Check sheet for the modelled part. Datum: model origin and axes. Units: mm. A direction names the side the tool comes from. Round coordinates to 2 decimals unless told otherwise and drop trailing zeros. Order: outer loops, then holes, each group sorted by start corner. A loop starts at its lowest first (then second) coordinate and runs counter-clockwise, first axis right, second up. Notation, with made-up numbers: (-40, -7) -> (7, -7) arc R19 cw to (7, 5) -> close; hole circle Ø2 at (86, 60.25). An arc over 180 degrees is marked (long way). Answer in a Markdown table with one row per item. Add a question column.
1. Access from +Z, -Z, +X, -X, +Y, -Y to the whole of each face (thin tool, end or side, straight path). Record for faces 5 (the flat face through (10, -120, 4)), 6 (the cylindrical face through (29.62, -151.84, 6.52)), 7 (the flat face through (40, -150, 4)).
2. Sectioned sample at C-C, the plane z = 1.25. Record the boundary of the cut face in (x, y), then the cut area to 3 significant figures.
3. Sectioned sample at A-A, the plane y = -145. Record the boundary of the cut face in (x, z), then the cut area to 3 significant figures.
4. Sectioned sample at B-B, the plane x = 32. Record the boundary of the cut face in (y, z).
5. Material ranges on L1, parallel to Y at x = 0, z = 5.7; L2, parallel to Y at x = 0, z = 3.05; L3, parallel to X at y = -125, z = 4.05, recorded low to high. Write a range as from..to.
6. Depth check by flat-ended pin: P1, Ø1.8, axis at x = -1, y = -145, coming from the +Z side; P2, Ø2.5, axis at y = -119.5, z = 3.5, coming from the +X side; P3, Ø3.5, axis at x = 0, y = -145, coming from the -Z side; P4, Ø4, axis at x = 29.5, z = 2.5, coming from the +Y side. Enter the tip coordinate at first touch or a pass-through.
7. Sectioned sample at D-D, the plane z = 6.75. Record the boundary of the cut face in (x, y), then the cut area to 3 significant figures.
8. Draft check along X on faces 1 (the flat face through (-10, -130, 4)), 2 (the flat face through (19.3, -151.3, 5)), 3 (the cylindrical face through (-0.35, -146.56, 2.46)), 4 (the flat face through (10, -140, 0)). Enter one of: +X half, -X half, draft (parallel to the pull), parting line (faces both ways), or undercut.
```python
from build123d import *

# Parameters (mm, degrees)
SKETCH_1_R          = 1.6
EXTRUDE_1_DEPTH     = 8
SKETCH_2_R          = 3
CUT_EXTRUDE_1_DEPTH = 3
FILLET_1_R          = 10


with BuildPart() as part:
    # 草图1 → 凸台-拉伸1 (new body)
    with BuildSketch(Plane.XY):
        Polygon((-10, -110), (10, -110), (10, -140.028839027), (40, -140.028839027), (40, -160), (-10, -160), align=None)
        with Locations((0, -125)):
            Circle(SKETCH_1_R, mode=Mode.SUBTRACT)
        with Locations((0, -145)):
            Circle(SKETCH_1_R, mode=Mode.SUBTRACT)
        with Locations((18, -150.014419513)):
            Circle(SKETCH_1_R, mode=Mode.SUBTRACT)
        with Locations((32, -150.014419513)):
            Circle(SKETCH_1_R, mode=Mode.SUBTRACT)
    extrude(amount=EXTRUDE_1_DEPTH)

    # 草图2 → 切除-拉伸1 (cut)
    with BuildSketch(Plane.XY.offset(8)):
        with Locations((32, -150.014419513)):
            Circle(SKETCH_2_R)
        with Locations((18, -150.014419513)):
            Circle(SKETCH_2_R)
        with Locations((0, -145)):
            Circle(SKETCH_2_R)
        with Locations((0, -125)):
            Circle(SKETCH_2_R)
    extrude(amount=-CUT_EXTRUDE_1_DEPTH, mode=Mode.SUBTRACT)

    # 圆角1
    fillet_1_edges = [part.edges().sort_by_distance(p)[0] for p in [
        (10, -140.028839027, 4),
        (-10, -160, 4),
    ]]
    fillet(fillet_1_edges, radius=FILLET_1_R)


solid = part.part
```
Answer key:
| question | item | result |
|---|---|---|
| 1 | face 5 | +Z, -Z, +X, +Y |
| 1 | face 6 | +Z |
| 1 | face 7 | +Z, -Z, +X, +Y, -Y |
| 2 | outline | (-10, -150) arc R10 ccw to (0, -160) -> (40, -160) -> (40, -140.03) -> (20, -140.03) arc R10 cw to (10, -130.03) -> (10, -110) -> (-10, -110) -> close; hole circle Ø3.2 at (0, -145); hole circle Ø3.2 at (0, -125); hole circle Ø3.2 at (18, -150.01); hole circle Ø3.2 at (32, -150.01) |
| 2 | area | 1,570 mm² |
| 3 | outline | (-10, 0) -> (-1.6, 0) -> (-1.6, 5) -> (-3, 5) -> (-3, 8) -> (-10, 8) -> close; (1.6, 0) -> (40, 0) -> (40, 8) -> (3, 8) -> (3, 5) -> (1.6, 5) -> close |
| 3 | area | 366 mm² |
| 4 | outline | (-160, 0) -> (-151.61, 0) -> (-151.61, 5) -> (-153.01, 5) -> (-153.01, 8) -> (-160, 8) -> close; (-148.41, 0) -> (-140.03, 0) -> (-140.03, 8) -> (-147.01, 8) -> (-147.01, 5) -> (-148.41, 5) -> close |
| 5 | L1 | y = -160..-148, -142..-128, -122..-110 |
| 5 | L2 | y = -160..-146.6, -143.4..-126.6, -123.4..-110 |
| 5 | L3 | x = -10..-1.6, 1.6..10 |
| 6 | P1 | stops at z = 5 |
| 6 | P2 | stops at x = 10 |
| 6 | P3 | stops at z = 0 |
| 6 | P4 | stops at y = -140.03 |
| 7 | outline | (-10, -150) arc R10 ccw to (0, -160) -> (40, -160) -> (40, -140.03) -> (20, -140.03) arc R10 cw to (10, -130.03) -> (10, -110) -> (-10, -110) -> close; hole circle Ø6 at (0, -145); hole circle Ø6 at (0, -125); hole circle Ø6 at (18, -150.01); hole circle Ø6 at (32, -150.01) |
| 7 | area | 1,490 mm² |
| 8 | face 1 | -X half |
| 8 | face 2 | undercut |
| 8 | face 3 | undercut |
| 8 | face 4 | draft |
